from build123d import *

# Parameters (mm, degrees)
SKETCH1_R           = 63.5
BOSS_EXTRUDE2_DEPTH = 25.4
SKETCH2_R           = 6.35
BOSS_EXTRUDE3_DEPTH = 50.8
BOSS_EXTRUDE4_START = 25.4
SKETCH3_R           = 63.5
BOSS_EXTRUDE4_DEPTH = 25.4
CUT_EXTRUDE2_START  = 50.8
SKETCH4_W           = 127
SKETCH4_H           = 101.6
CUT_EXTRUDE2_DEPTH  = 76.2
SKETCH5_R           = 50.8
BOSS_EXTRUDE5_DEPTH = 12.7
SKETCH6_R           = 6.35
BOSS_EXTRUDE6_DEPTH = 25.4


with BuildPart() as part:
    # Sketch1 → Boss-Extrude2 (new body)
    with BuildSketch(Plane.XY):
        Circle(SKETCH1_R)
    extrude(amount=BOSS_EXTRUDE2_DEPTH)

    # Sketch2 → Boss-Extrude3 (add)
    with BuildSketch(Plane(origin=(0, 0, 0), x_dir=(-1, 0, 0), z_dir=(0, 0, -1))):
        with Locations(Location((0, 0, 0), (0, 0, 180))):
            Circle(SKETCH2_R)
    extrude(amount=BOSS_EXTRUDE3_DEPTH)

    # Sketch3 → Boss-Extrude4 (add)
    with BuildSketch(Plane(origin=(0, 0, -50.8), x_dir=(-1, 0, 0), z_dir=(0, 0, -1)).offset(BOSS_EXTRUDE4_START)):
        with Locations(Location((0, 0, 0), (0, 0, 180))):
            Circle(SKETCH3_R)
    extrude(amount=-BOSS_EXTRUDE4_DEPTH)

    # Sketch4 → Cut-Extrude2 (cut)
    with BuildSketch(Plane(origin=(0, 0, 0), x_dir=(1, 0, 0), z_dir=(0, 1, 0)).offset(CUT_EXTRUDE2_START)):
        with Locations((0, 25.4)):
            Rectangle(SKETCH4_W, SKETCH4_H)
    extrude(amount=CUT_EXTRUDE2_DEPTH, mode=Mode.SUBTRACT)

    # Sketch5 → Boss-Extrude5 (add)
    with BuildSketch(Plane(origin=(0, 50.8, 0), x_dir=(1, 0, 0), z_dir=(0, 1, 0))):
        with Locations(Location((0, 25.4, 0), (0, 0, 270))):
            Circle(SKETCH5_R)
    extrude(amount=BOSS_EXTRUDE5_DEPTH)

    # Sketch6 → Boss-Extrude6 (add)
    with BuildSketch(Plane(origin=(0, 63.5, 0), x_dir=(1, 0, 0), z_dir=(0, 1, 0))):
        with Locations(Location((0, 25.4, 0), (0, 0, 270))):
            Circle(SKETCH6_R)
    extrude(amount=BOSS_EXTRUDE6_DEPTH)


solid = part.part
For this review, take the finished solid that the model builds, in its own axes (mm). A direction names the side the tool comes from. Round coordinates to 2 decimals unless told otherwise and drop trailing zeros. Order: outer loops, then holes, each group sorted by start corner. A loop starts at its lowest first (then second) coordinate and runs counter-clockwise, first axis right, second up. Notation, with made-up numbers: (44.5, 68.5) -> (75.5, 68.5) arc R8 ccw to (75.5, 80.5) -> close; hole circle Ø5 at (-25, -4.5). An arc over 180 degrees is marked (long way). Write item = value, one per line. Start each with the question number.
1) Take a section at A-A on z = -25.4. State the section outline as (x, y) points, plus the area to 3 significant figures.
2) Take a section at C-C on x = 43.5. State the section outline as (y, z) points.
3) Take a section at D-D on y = 0. State the section outline as (x, z) points.
4) Tool access review of faces 4 (the face through (-29, 50.8, 20)), 5 (the face through (29, 50.8, -71)), 6 (the face through (15.259, 57.061, 23.054)): name each direction out of +Z, -Z, +X, -X, +Y, -Y from which nothing blocks a thin tool from reaching the whole face with its end or side.
5) The part is to be moulded in two halves that separate along Y. For faces 1 (the face through (29, 50.8, 20)), 2 (the face through (-1, -6, 25.4)), 3 (the face through (2.93, 5.634, -25.044)), say which applies: +Y half, -Y half, draft (parallel to the pull), parting line (faces both ways), or undercut.
6) Take a section at B-B on y = 36.5. State the section outline as (x, z) points.
7) Insertion check: pin 1 (19 mm diameter, centred on x = -13.5, z = 15.5, fed in from +Y); pin 2 (12 mm diameter, centred on y = -40, z = -7, fed in from -X); pin 3 (5 mm diameter, centred on x = -24, z = -25, fed in from -Y); pin 4 (2 mm diameter, centred on y = -9.5, z = 5.5, fed in from -X). Each pin has a flat end and moves straight along its axis. Give the tip position at first contact, or say it passes through.
8) To check wall thickness, follow line 1 (Z direction, x = -9, y = -26); line 2 (Y direction, x = -31, z = -42); line 3 (Y direction, x = 16.5, z = -51.5). State the ranges of each line that lie inside material, in increasing order. Write a range as from..to.
Verdict:
q1.outline = (-50.8, 50.8) -> (50.8, 50.8) -> (50.8, 63.5) -> (6.35, 63.5) -> (6.35, 88.9) -> (-6.35, 88.9) -> (-6.35, 63.5) -> (-50.8, 63.5) -> close; circle Ø12.7 at (0, 0)
q1.area = 1,740 mm2
q2.outline = (-46.26, -76.2) -> (46.26, -76.2) -> (46.26, -50.8) -> (-46.26, -50.8) -> close; (-46.26, 0) -> (46.26, 0) -> (46.26, 25.4) -> (-46.26, 25.4) -> close; (50.8, -51.64) -> (63.5, -51.64) -> (63.5, 0.84) -> (50.8, 0.84) -> close
q3.outline = (-63.5, -76.2) -> (63.5, -76.2) -> (63.5, -50.8) -> (6.35, -50.8) -> (6.35, 0) -> (63.5, 0) -> (63.5, 25.4) -> (-63.5, 25.4) -> (-63.5, 0) -> (-6.35, 0) -> (-6.35, -50.8) -> (-63.5, -50.8) -> close
q4.face_4 = +Z, -X, +Y
q4.face_5 = -Z, +X, +Y
q4.face_6 = +Y
q5.face_1 = +Y half
q5.face_2 = draft
q5.face_3 = undercut
q6.outline = (-51.96, -76.2) -> (51.96, -76.2) -> (51.96, -50.8) -> (-51.96, -50.8) -> close; (-51.96, 0) -> (51.96, 0) -> (51.96, 25.4) -> (-51.96, 25.4) -> close
q7.pin_1 = 63.5
q7.pin_2 = through
q7.pin_3 = 50.8
q7.pin_4 = -62.93
q8.line_1 = -76.2..-50.8, 0..25.4
q8.line_2 = 50.8..63.5
q8.line_3 = -61.32..63.5
